Drawing for the job (mm, zero at the part's lowest x, y, z). A direction names the side the tool comes from. Coordinates: 2 decimals unless noted, no trailing zeros. Order: outer loops, then holes, each group sorted by start corner. A loop starts at its lowest first (then second) coordinate and runs counter-clockwise, first axis right, second up.
1) Cut at A-A (x = 7.75). List the corners of the cut face in (y, z), and give its area (3 significant figures).
2) Tool access for the marked faces 4 and 5: list every direction of +Z, -Z, +X, -X, +Y, -Y with a clear straight run to the whole face (end or side of a thin tool).
3) Cut at B-B (y = 12.7). Give the number of separate pieces and of enclosed holes in the cut face, and give its area (3 significant figures).
4) Pin check, flat tips, straight feed: pin 1 Ø8 at (x, y) = (19, 13.5) entering from -Z; pin 2 Ø3.5 at (x, y) = (17.5, 12.5) entering from +Z; pin 3 Ø1 at (x, y) = (12, 4) entering from -Z. Stop position of each tip, or through.
5) Mould opens along Z. For the marked faces 1, 2 and 3 say: +Z half, -Z half, draft (parallel to the pull), parting line (faces both ways), or undercut.
6) Wall check: L1, parallel to X at y = 12.7, z = 22.3 (1 decimal); L2, parallel to Z at x = 17.5, y = 10; L3, parallel to Y at x = 23, z = 12.5 (1 decimal). Give the ranges that are in metal, low to high.
7) Cut at D-D (z = 8.5). List the corners of the cut face in (x, y) (1 decimal).
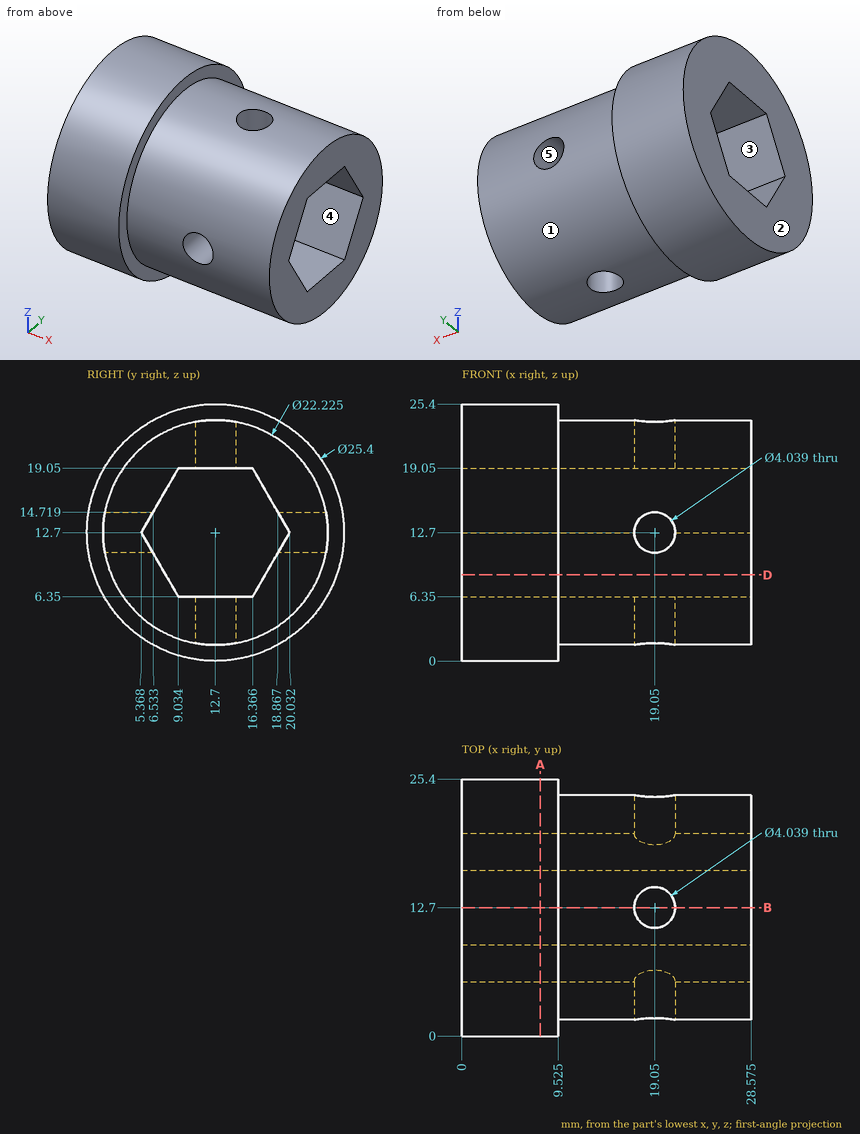
Geometry check:
1. outline: circle Ø25.4 at (12.7, 12.7); hole (5.37, 12.7) - (9.03, 6.35) - (16.37, 6.35) - (20.03, 12.7) - (16.37, 19.05) - (9.03, 19.05) - close
1. area: 367 mm2
2. face 4: +X, -X
2. face 5: +Y, -Y
3. separate pieces: 4
3. enclosed holes: 0
3. area: 264 mm2
4. pin 1: stops at z = 1.59
4. pin 2: stops at z = 23.81
4. pin 3: stops at z = 5.2
5. face 1: parting line
5. face 2: draft
5. face 3: undercut
6. L1: x = 0 to 17, 21.1 to 28.6
6. L2: z = 1.92 to 6.35, 19.05 to 23.48
6. L3: y = 1.6 to 5.5, 19.9 to 23.8
7. outline: (0, 0.7) - (9.5, 0.7) - (9.5, 2.4) - (28.6, 2.4) - (28.6, 7.8) - (0, 7.8) - close; (0, 17.6) - (28.6, 17.6) - (28.6, 23) - (9.5, 23) - (9.5, 24.7) - (0, 24.7) - close
